from build123d import *

# Parameters (mm, degrees)
SKETCH2_W                           = 10
SKETCH2_H                           = 25
F_5_6_5_6_DIAMETER_HOLE1_AT_2_COUNT = 2
F_5_6_5_6_DIAMETER_HOLE1_AT_2_PITCH = 17.5
F_5_6_5_6_DIAMETER_HOLE1_AT_3_COUNT = 2
F_5_6_5_6_DIAMETER_HOLE1_AT_3_PITCH = 30.310889132
F_5_6_5_6_DIAMETER_HOLE1_AT_4_COUNT = 2
F_5_6_5_6_DIAMETER_HOLE1_AT_4_PITCH = 35
F_5_6_5_6_DIAMETER_HOLE1_AT_5_COUNT = 2
F_5_6_5_6_DIAMETER_HOLE1_AT_5_PITCH = 30.310889132
F_5_6_5_6_DIAMETER_HOLE1_AT_6_COUNT = 2
F_5_6_5_6_DIAMETER_HOLE1_AT_6_PITCH = 17.5


with BuildPart() as part:
    # Sketch2 → Revolve1 (revolve)
    with BuildSketch(Plane.XY, mode=Mode.PRIVATE) as revolve1_sk:
        with Locations((17.5, 12.5)):
            Rectangle(SKETCH2_W, SKETCH2_H)
    revolve1 = revolve(revolve1_sk.sketch.rotate(Axis((0, 0, 0), (0, 1, 0)), 90), axis=Axis((0, 0, 0), (0, 1, 0)))

    # Sketch5 → Ø5.6 (5.6) Diameter Hole1 (revolve, cut)
    with BuildSketch(Plane(origin=(15.155444566, 25, 8.75), x_dir=(0, 0, 1), z_dir=(1, 0, 0))):
        Polygon((0, 0), (0, 9.682409733), (2.8, 8), (2.8, 0), align=None)
    f_5_6_5_6_diameter_hole1 = revolve(axis=Axis((15.155444566, 31.35, 8.75), (0, -1, 0)), mode=Mode.SUBTRACT)

    # Ø5.6 (5.6) Diameter Hole1 at 2: Ø5.6 (5.6) Diameter Hole1 ×2
    with Locations(*[Vector(-0.8660254037844417, 0, 0.49999999999999495) * (i * F_5_6_5_6_DIAMETER_HOLE1_AT_2_PITCH) for i in range(1, F_5_6_5_6_DIAMETER_HOLE1_AT_2_COUNT)]):
        add(f_5_6_5_6_diameter_hole1, mode=Mode.SUBTRACT)

    # Ø5.6 (5.6) Diameter Hole1 at 3: Ø5.6 (5.6) Diameter Hole1 ×2
    with Locations(*[(-i * F_5_6_5_6_DIAMETER_HOLE1_AT_3_PITCH, 0, 0) for i in range(1, F_5_6_5_6_DIAMETER_HOLE1_AT_3_COUNT)]):
        add(f_5_6_5_6_diameter_hole1, mode=Mode.SUBTRACT)

    # Ø5.6 (5.6) Diameter Hole1 at 4: Ø5.6 (5.6) Diameter Hole1 ×2
    with Locations(*[Vector(-0.8660254037844346, 0, -0.5000000000000072) * (i * F_5_6_5_6_DIAMETER_HOLE1_AT_4_PITCH) for i in range(1, F_5_6_5_6_DIAMETER_HOLE1_AT_4_COUNT)]):
        add(f_5_6_5_6_diameter_hole1, mode=Mode.SUBTRACT)

    # Ø5.6 (5.6) Diameter Hole1 at 5: Ø5.6 (5.6) Diameter Hole1 ×2
    with Locations(*[Vector(-0.49999999999999195, 0, -0.8660254037844433) * (i * F_5_6_5_6_DIAMETER_HOLE1_AT_5_PITCH) for i in range(1, F_5_6_5_6_DIAMETER_HOLE1_AT_5_COUNT)]):
        add(f_5_6_5_6_diameter_hole1, mode=Mode.SUBTRACT)

    # Ø5.6 (5.6) Diameter Hole1 at 6: Ø5.6 (5.6) Diameter Hole1 ×2
    with Locations(*[(0, 0, -i * F_5_6_5_6_DIAMETER_HOLE1_AT_6_PITCH) for i in range(1, F_5_6_5_6_DIAMETER_HOLE1_AT_6_COUNT)]):
        add(f_5_6_5_6_diameter_hole1, mode=Mode.SUBTRACT)

    # Mirror1: Revolve1, Ø5.6 (5.6) Diameter Hole1 across plane
    add(revolve1.mirror(Plane.ZX))
    add(f_5_6_5_6_diameter_hole1.mirror(Plane.ZX), mode=Mode.SUBTRACT)

    # Mirror1 copy 1 sketch → Mirror1 copy 1 (revolve, cut)
    with BuildSketch(Plane(origin=(0, -25, 17.5), x_dir=(0, 0, 1), z_dir=(1, 0, 0))):
        Polygon((0, 0), (0, -9.682409733), (2.8, -8), (2.8, 0), align=None)
    revolve(axis=Axis((0, -31.35, 17.5), (0, -1, 0)), mode=Mode.SUBTRACT)

    # Mirror1 copy 2 sketch → Mirror1 copy 2 (revolve, cut)
    with BuildSketch(Plane(origin=(-15.155444566, -25, 8.75), x_dir=(0, 0, 1), z_dir=(1, 0, 0))):
        Polygon((0, 0), (0, -9.682409733), (2.8, -8), (2.8, 0), align=None)
    revolve(axis=Axis((-15.155444566, -31.35, 8.75), (0, -1, 0)), mode=Mode.SUBTRACT)

    # Mirror1 copy 3 sketch → Mirror1 copy 3 (revolve, cut)
    with BuildSketch(Plane(origin=(-15.155444566, -25, -8.75), x_dir=(0, 0, 1), z_dir=(1, 0, 0))):
        Polygon((0, 0), (0, -9.682409733), (2.8, -8), (2.8, 0), align=None)
    revolve(axis=Axis((-15.155444566, -31.35, -8.75), (0, -1, 0)), mode=Mode.SUBTRACT)

    # Mirror1 copy 4 sketch → Mirror1 copy 4 (revolve, cut)
    with BuildSketch(Plane(origin=(0, -25, -17.5), x_dir=(0, 0, 1), z_dir=(1, 0, 0))):
        Polygon((0, 0), (0, -9.682409733), (2.8, -8), (2.8, 0), align=None)
    revolve(axis=Axis((0, -31.35, -17.5), (0, -1, 0)), mode=Mode.SUBTRACT)

    # Mirror1 copy 5 sketch → Mirror1 copy 5 (revolve, cut)
    with BuildSketch(Plane(origin=(15.155444566, -25, -8.75), x_dir=(0, 0, 1), z_dir=(1, 0, 0))):
        Polygon((0, 0), (0, -9.682409733), (2.8, -8), (2.8, 0), align=None)
    revolve(axis=Axis((15.155444566, -31.35, -8.75), (0, -1, 0)), mode=Mode.SUBTRACT)


solid = part.part
Input: part model. Units: mm. Frame: model coordinates. A direction names the side the tool comes from. Coordinates: 2 decimals unless noted, no trailing zeros. Order: outer loops, then holes, each group sorted by start corner. A loop starts at its lowest first (then second) coordinate and runs counter-clockwise, first axis right, second up.
1. Cut plane C-C, the plane y = 13.5. Return loops of the section in (x, z).
Checked values:
outline: circle Ø45 at (0, 0); hole circle Ø25 at (0, 0)
2. Cut plane D-D, the plane x = 19. Return loops of the section in (y, z).
Checked values:
outline: (-25, -12.05) - (25, -12.05) - (25, 12.05) - (-25, 12.05) - close
3. Draft query along X for faces 3 (the flat face through (10, 25, 10)), 4 (the cylindrical face through (-0.84, 21.06, -14.83)). Return one class per face: +X half, -X half, draft (parallel to the pull), parting line (faces both ways), or undercut.
Checked values:
face 3: draft
face 4: undercut
4. Contact query for flat-ended pins moving along their axis: P1, Ø15, axis at x = 0, z = 0, coming from the -Y side; P2, Ø1.5, axis at x = 1.5, y = -6.5, coming from the -Z side; P3, Ø4, axis at x = -9.5, y = -10.5, coming from the +Z side; P4, Ø5, axis at x = 0, z = 17.5, coming from the +Y side. Output: stop coordinate, or through.
Checked values:
P1: passes through
P2: stops at z = -22.49
P3: stops at z = 21.21
P4: stops at y = 16.82
5. Ray query, line 1 along X through (y, z) = (8, 0); line 2 along X through (y, z) = (-20, 8); line 3 along X through (y, z) = (-21.5, 10.5). Return the intervals inside material, ascending.
Checked values:
line 1: x = -22.5 to -12.5, 12.5 to 22.5
line 2: x = -21.03 to -17.85, -12.46 to -9.6, 9.6 to 12.46, 17.85 to 21.03
line 3: x = -19.9 to -17.34, -12.97 to -6.78, 6.78 to 12.97, 17.34 to 19.9
6. Access query for faces 1 (the cylindrical face through (-0.1, -21.1, 14.7)), 2 (the cylindrical face through (-2.36, 21.06, 19.01)). Directions: +Z, -Z, +X, -X, +Y, -Y. A direction counts if a zero-diameter tool reaches every point of the face in a straight line with its end or side. Return the directions, or none.
Checked values:
face 1: -Y
face 2: +Y
7. Cut plane B-B, the plane y = -20. Return loops of the section in (x, z), plus the area to 3 significant figures.
Checked values:
outline: circle Ø45 at (0, 0); hole circle Ø5.6 at (-15.16, -8.75); hole circle Ø5.6 at (-15.16, 8.75); hole circle Ø25 at (0, 0); hole circle Ø5.6 at (0, -17.5); hole circle Ø5.6 at (0, 17.5); hole circle Ø5.6 at (15.16, -8.75); hole circle Ø5.6 at (15.16, 8.75)
area: 952 mm2
8. Cut plane A-A, the plane x = 3.5. Return loops of the section in (y, z).
Checked values:
outline: (-25, -22.23) - (25, -22.23) - (25, -12) - (-25, -12) - close; (-25, 12) - (25, 12) - (25, 22.23) - (-25, 22.23) - close
